Autodesk Fusion 360 part; units mm, degrees
sketch "Esquisse1" plane through (0, 0, 0) normal (0, 0, 1) x (1, 0, 0)
  line L0 (-75, 95) -> (75, 95)
  line L1 (75, 95) -> (75, -60)
  line L2 (75, -60) -> (-75, -60)
  line L3 (-75, -60) -> (-75, 95)
  line L4 (0, 1.75) -> (0, 22.5)
  line L5 (1.75, 0) -> (22.5, 0)
  line L6 (20, 0) -> (2.5, 0)
  dimension "d1" = 150
  dimension "d2" = 155
  dimension "d69" = 95
extrude "Extrusion1" add sketch "Esquisse1" against normal blind 25
sketch "Esquisse2" plane through (0, 0, 0) normal (0, 0, 1) x (-1, 0, 0)
  line L0 (75, 60) -> (-75, 60)
  line L1 (-75, 60) -> (-75, -95)
  line L2 (-75, -95) -> (75, -95)
  line L3 (75, -95) -> (75, 60)
  circle A0 centre (0, 0) radius 11.125
  dimension "d5" = 22.25
extrude "Extrusion2" cut sketch "Esquisse2" against normal blind 12 contours A0
sketch "Esquisse3" plane through (0, 0, -25) normal (0, 0, -1) x (1, 0, 0)
  line L0 (75, 60) -> (-75, 60)
  line L1 (-75, 60) -> (-75, -95)
  line L2 (-75, -95) -> (75, -95)
  line L3 (75, -95) -> (75, 60)
sketch "Esquisse4" plane through (0, 0, -25) normal (0, 0, -1) x (1, 0, 0)
  circle A0 centre (0, 0) radius 11.125
  dimension "d8" = 22.25
extrude "Extrusion3" cut sketch "Esquisse4" against normal blind 10
sketch "Esquisse5" plane through (0, 0, -12) normal (0, 0, 1) x (-1, 0, 0)
  circle A0 centre (0, 0) radius 11.125
  circle A1 centre (0, 0) radius 4
  dimension "d11" = 8
extrude "Extrusion4" cut sketch "Esquisse5" against normal blind 51 contours A1
sketch "Esquisse6" plane through (0, 0, 0) normal (0, 0, 1) x (-1, 0, 0)
  circle A0 centre (0, 0) radius 11.125
  line L0 (75, 60) -> (-75, 60)
  line L1 (-75, 60) -> (-75, -95)
  line L2 (-75, -95) -> (75, -95)
  line L3 (75, -95) -> (75, 60)
  line L4 (-21.1, -45) -> (21.1, -45)
  line L5 (21.1, -45) -> (21.1, -87.2)
  line L6 (21.1, -87.2) -> (-21.1, -87.2)
  line L7 (-21.1, -87.2) -> (-21.1, -45)
  line L8 (-20, 0) -> (-2.5, 0)
  line L9 (0, -1.75) -> (0, -22.5)
  dimension "d14" = 45
  dimension "d15" = 42.2
  dimension "d16" = 42.2
extrude "Extrusion5" cut sketch "Esquisse6" against normal blind 17 contours L4 L5 L6 L7
fillet "Congé1" radius 3 4 edges at (21.1, 87.2, -8.5) (21.1, 45, -8.5) (-21.1, 87.2, -8.5) (-21.1, 45, -8.5)
sketch "Esquisse7" plane through (0, 0, -17) normal (0, 0, 1) x (-1, 0, 0)
  arc A0 (21.1, -48) -> (18.1, -45) centre (18.1, -48) ccw
  line L0 (18.1, -45) -> (-18.1, -45)
  arc A1 (-18.1, -45) -> (-21.1, -48) centre (-18.1, -48) ccw
  line L1 (-21.1, -48) -> (-21.1, -84.2)
  line L2 (21.1, -84.2) -> (21.1, -48)
  circle A2 centre (0, -66.1) radius 11.1
  line L3 (21.1, -48) -> (21.1, -84.2)
  line L4 (18.1, -87.2) -> (-18.1, -87.2)
  arc A3 (-21.1, -84.2) -> (-18.1, -87.2) centre (-18.1, -84.2) ccw
  line L5 (-18.1, -87.2) -> (18.1, -87.2)
  arc A4 (18.1, -87.2) -> (21.1, -84.2) centre (18.1, -84.2) ccw
  dimension "d21" = 22.2
  dimension "d22" = 21.1
  dimension "d23" = 21.1
extrude "Extrusion6" cut sketch "Esquisse7" against normal blind 2.5 contours A2
sketch "Esquisse8" plane through (0, 0, -19.5) normal (0, 0, 1) x (-1, 0, 0)
  circle A0 centre (0, -66.1) radius 3
  circle A1 centre (0, -66.1) radius 11.1
  circle A2 centre (0, -66.1) radius 11.1
  dimension "d26" = 6
extrude "Extrusion7" cut sketch "Esquisse8" against normal blind 33 contours A0
sketch "Esquisse9" plane through (0, 0, -17) normal (0, 0, 1) x (-1, 0, 0)
  arc A0 (21.1, -48) -> (18.1, -45) centre (18.1, -48) ccw
  line L0 (18.1, -45) -> (-18.1, -45)
  arc A1 (-18.1, -45) -> (-21.1, -48) centre (-18.1, -48) ccw
  line L1 (-21.1, -48) -> (-21.1, -84.2)
  line L2 (21.1, -84.2) -> (21.1, -48)
  circle A2 centre (0, -66.1) radius 11.1
  arc A3 (-21.1, -84.2) -> (-18.1, -87.2) centre (-18.1, -84.2) ccw
  line L3 (-18.1, -87.2) -> (18.1, -87.2)
  arc A4 (18.1, -87.2) -> (21.1, -84.2) centre (18.1, -84.2) ccw
  point P0 (-15.5, -50.6)
  point P1 (15.5, -50.6)
  point P2 (-15.5, -81.6)
  point P3 (15.5, -81.6)
  dimension "d29" = 15.5
  dimension "d30" = 15.5
  dimension "d33" = 31
  dimension "d34" = -31
hole "Perçage1" at (15.5, 50.6, -17) at (-15.5, 50.6, -17) at (-15.5, 81.6, -17) at (15.5, 81.6, -17) direction (0, 0, -1) diameter 4 depth 30 tip angle 118
mirror "Symétrie miroir1" [suppressed]
sketch "Esquisse10" plane through (0, 0, -25) normal (0, 0, -1) x (1, 0, 0)
  line L0 (1.75, 0) -> (22.5, 0)
  line L1 (0, -1.75) -> (0, -22.5)
  line L2 (0, -2.5) -> (0, -20)
  line L3 (20, 0) -> (2.5, 0)
  line L4 (-75, -95) -> (75, -95)
  line L5 (-75, 60) -> (-75, -95)
  point P0 (-63, -83)
  dimension "d74" = 12
  dimension "d75" = 12
hole "Perçage2" at (-63, 83, -25) direction (0, 0, 1) diameter 5 depth 30 tip angle 118
sketch "Esquisse11" plane through (-75, 0, 0) normal (-1, 0, 0) x (0, -1, 0)
  line L0 (60, 0) -> (-95, 0)
  line L1 (-95, 0) -> (-95, -25)
  line L2 (-95, -25) -> (60, -25)
  line L3 (60, -25) -> (60, 0)
  circle A0 centre (-35, -12.5) radius 4.125
  line L4 (60, -25) -> (-95, -25)
  line L5 (0, 2.5) -> (0, 20)
  dimension "d49" = 8.25
  dimension "d50" = 12.5
  dimension "d51" = 35
extrude "Extrusion8" cut sketch "Esquisse11" against normal blind 165 contours A0
mirror "Symétrie miroir2" about plane through (0, 0, 0) normal (0, 1, 0) of "Extrusion8"
sketch "Esquisse12" plane through (0, 0, -25) normal (0, 0, -1) x (1, 0, 0)
sketch "Esquisse13" plane through (0, 0, -25) normal (0, 0, -1) x (1, 0, 0)
sketch "Esquisse14" plane through (0, 0, -25) normal (0, 0, -1) x (1, 0, 0)
  arc A0 (55, 19.2) -> (55, 15) centre (55, 17.1) ccw
  line L0 (55, 19.2) -> (63, 19.2)
  arc A1 (63, 15) -> (63, 19.2) centre (63, 17.1) ccw
  line L1 (55, 15) -> (63, 15)
  line L2 (0, -1.75) -> (0, -22.5)
  line L3 (1.75, 0) -> (22.5, 0)
  line L4 (0, -2.5) -> (0, -20)
  dimension "d57" = 8
  dimension "d60" = 4.2
  dimension "d70" = 15
  dimension "d71" = 55
extrude "Extrusion9" cut sketch "Esquisse14" against normal blind 35
pattern_linear "Réseau R1" count 2 spacing 31 along (0, -1, 0) count 2 spacing 31 along (-1, 0, 0) of "Extrusion9"
sketch "Esquisse15" plane through (0, 0, 0) normal (0, 0, 1) x (-1, 0, 0)
  line L0 (-24, 46) -> (-32, 46)
  arc A0 (-32, 50.2) -> (-32, 46) centre (-32, 48.1) ccw
  line L1 (-32, 50.2) -> (-24, 50.2)
  arc A1 (-24, 46) -> (-24, 50.2) centre (-24, 48.1) ccw
  line L2 (-24, 15) -> (-32, 15)
  arc A2 (-32, 19.2) -> (-32, 15) centre (-32, 17.1) ccw
  line L3 (-32, 19.2) -> (-24, 19.2)
  arc A3 (-24, 15) -> (-24, 19.2) centre (-24, 17.1) ccw
  line L4 (-55, 46) -> (-63, 46)
  arc A4 (-63, 50.2) -> (-63, 46) centre (-63, 48.1) ccw
  line L5 (-63, 50.2) -> (-55, 50.2)
  arc A5 (-55, 46) -> (-55, 50.2) centre (-55, 48.1) ccw
  line L6 (-55, 15) -> (-63, 15)
  arc A6 (-63, 19.2) -> (-63, 15) centre (-63, 17.1) ccw
  line L7 (-63, 19.2) -> (-55, 19.2)
  arc A7 (-55, 15) -> (-55, 19.2) centre (-55, 17.1) ccw
  circle A8 centre (63, -83) radius 2.5
  line L8 (21.1, -48) -> (21.1, -84.2)
  arc A9 (18.1, -87.2) -> (21.1, -84.2) centre (18.1, -84.2) ccw
  line L9 (18.1, -87.2) -> (-18.1, -87.2)
  arc A10 (-21.1, -84.2) -> (-18.1, -87.2) centre (-18.1, -84.2) ccw
  line L10 (-21.1, -84.2) -> (-21.1, -48)
  arc A11 (-18.1, -45) -> (-21.1, -48) centre (-18.1, -48) ccw
  line L11 (-18.1, -45) -> (18.1, -45)
  arc A12 (21.1, -48) -> (18.1, -45) centre (18.1, -48) ccw
  circle A13 centre (0, 0) radius 11.125
  line L12 (75, 60) -> (-75, 60)
  line L13 (-75, 60) -> (-75, -95)
  line L14 (-75, -95) -> (75, -95)
  line L15 (75, -95) -> (75, 60)
  point P0 (63, 48)
  dimension "d76" = 12
  dimension "d77" = 12
hole "Perçage3" at (-63, -48, 0) direction (0, 0, -1) diameter 5 depth 50 tip angle 118
fillet "Congé2" radius 10 1 edges at (-75, 95, -12.5)
fillet "Congé2" radius 10 3 edges at (75, 95, -12.5) (75, -60, -12.5) (-75, -60, -12.5)
sketch "Esquisse16" plane through (0, 0, -25) normal (0, 0, -1) x (1, 0, 0)
sketch "Esquisse17" plane through (0, 0, -25) normal (0, 0, -1) x (1, 0, 0)
  circle A0 centre (-63, 48) radius 10.25
  line L0 (75, 60) -> (-75, 60)
  line L1 (-75, 60) -> (-75, -95)
  dimension "d85" = 20.5
  dimension "d86" = 12
  dimension "d87" = 12
extrude "Extrusion10" cut sketch "Esquisse17" against normal blind 1
sketch "Esquisse18" plane through (0, 0, -25) normal (0, 0, -1) x (1, 0, 0)
  circle A0 centre (-63, -83) radius 10.25
  line L0 (-75, 60) -> (-75, -95)
  line L1 (-75, -95) -> (75, -95)
  dimension "d90" = 20.5
  dimension "d91" = 12
  dimension "d92" = 12
extrude "Extrusion11" cut sketch "Esquisse18" against normal blind 1
equation "d22 = ( 42.2 / 2 ) * 1 mm"
equation "d23 = ( 42.2 / 2 ) * 1 mm"
equation "d29 = ( 31 / 2 ) * 1 mm"
equation "d30 = ( 31 / 2 ) * 1 mm"
equation "d50 = ( 25 / 2 ) * 1 mm"
Work out the finished part from the listing and answer in its coordinate system (mm). A direction names the side the tool comes from. Coordinates: 2 decimals unless noted, no trailing zeros. Order: outer loops, then holes, each group sorted by start corner. A loop starts at its lowest first (then second) coordinate and runs counter-clockwise, first axis right, second up. Notation, with made-up numbers: (-9, 65.25) - (8, 65.25) arc R33 cw to (8, 95.25) - close; hole circle Ø1 at (-11, 3). An arc over 180 degrees is marked (long way). Answer as a JSON object with one key per item and string values.
1. Find section D-D on x = -38. Determine the outline of the cut face in (y, z) (3 decimals).
Output values:
{"outline": "(-60, -25) - (95, -25) - (95, 0) - (-60, 0) - close; hole circle Ø8.25 at (-35, -12.5); hole circle Ø8.25 at (35, -12.5)"}
2. Each of these flat-tipped pins is pushed along its axis until it touches: P1, Ø8, axis at x = -63, y = 83, coming from the -Z side; P2, Ø4.5, axis at x = 15.5, y = 50.6, coming from the +Z side; P3, Ø3, axis at x = 15.5, y = 81.6, coming from the -Z side; P4, Ø13.5, axis at x = 0, y = 0, coming from the -Z side. Where does it stop, or does it pass through?
Output values:
{"P1": "stops at z = -24", "P2": "stops at z = -17", "P3": "passes through", "P4": "stops at z = -15"}
3. The mould has two halves that part along X. Classify faces 1 (the face through (0, 5, -12)), 2 (the face through (71.99, 92.15, -12.68)), 3 (the face through (-1, 19, 0)): +X half, -X half, draft (parallel to the pull), parting line (faces both ways), or undercut.
Output values:
{"face 1": "undercut", "face 2": "+X half", "face 3": "draft"}
4. Find section C-C on z = -21.25. Count the separate pieces of the cut face and the enclosed holes in it, plus the area to 3 significant figures.
Output values:
{"separate pieces": "1", "enclosed holes": "12", "area": "22,500 mm²"}
5. Find section A-A on x = 15.5. Determine the outline of the cut face in (y, z) (3 decimals).
Output values:
{"outline": "(-60, -25) - (48.6, -25) - (48.6, -17) - (45, -17) - (45, 0) - (-60, 0) - close; (52.6, -25) - (79.6, -25) - (79.6, -17) - (52.6, -17) - close; (83.6, -25) - (95, -25) - (95, 0) - (87.2, 0) - (87.2, -17) - (83.6, -17) - close; hole circle Ø8.25 at (-35, -12.5); hole circle Ø8.25 at (35, -12.5)"}
6. A tool of negligible diameter and unlimited length cuts with its end or side. For faces 4 (the face through (59, -15, -13)), 5 (the face through (-9, 75, -17)), 6 (the face through (-61, -46, -24)), from which of +Z, -Z, +X, -X, +Y, -Y can it reach the whole face along a straight path? Write none if from no direction.
Output values:
{"face 4": "+Z, -Z", "face 5": "+Z", "face 6": "-Z"}
7. Consider line 1 (Y direction, x = 62.5, z = -16.75); line 2 (Y direction, x = 0, z = -18) (3 decimals); line 3 (Y direction, x = 0, z = -12.7). Determine where each line is inside the solid, lowest interval first.
Output values:
{"line 1": "y = -60 to -50.2, -46 to -19.2, -15 to 95", "line 2": "y = -60 to -11.125, 11.125 to 55, 77.2 to 95", "line 3": "y = -60 to -39.12, -30.88 to -4, 4 to 30.88, 39.12 to 45, 87.2 to 95"}
8. Find section B-B on y = -17.1. Determine the outline of the cut face in (x, z).
Output values:
{"outline": "(-75, -25) - (21.9, -25) - (21.9, 0) - (-75, 0) - close; (34.1, -25) - (52.9, -25) - (52.9, 0) - (34.1, 0) - close; (65.1, -25) - (75, -25) - (75, 0) - (65.1, 0) - close"}
